Job drawing, mm, ordinate dimensions from the low corner. One solid piece. A direction names the side the tool comes from. Round coordinates to 2 decimals unless told otherwise and drop trailing zeros. Loops run counter-clockwise (first coordinate to the right, second up) from the corner with the lowest first, then second, coordinate; pieces in that order, holes last. Notation, with made-up numbers: M 34.5,62.5 L 39.5,62.5 A36 ccw 39.5,99.5 Z; hole C 13,17.5 d11. An arc over 180 degrees is marked long. Use a Markdown table: item, result. Add a question column.
(1) Flat gauge pins, fed straight in: P1, Ø4, axis at x = 19.5, z = 8, coming from the +Y side; P2, Ø2, axis at y = 6, z = 11.5, coming from the +X side; P3, Ø3, axis at x = 25, z = 10.5, coming from the +Y side; P4, Ø1.5, axis at x = 30, z = 9.5, coming from the -Y side. Where does each tip first touch, or does it go through?
(2) Which spindle directions (+Z, -Z, +X, -X, +Y, -Y) get a long thin tool onto all of the face, cutting with end or side? Do the marked faces 1, 2, 3 and 4. Say none if no direction does.
(3) Band-saw the part on A-A, the plane z = 3.75. Write the cut outline in (x, y).
(4) Band-saw the part on B-B, the plane y = 19.75. Write the cut outline in (x, z).
(5) Wall check: L1, parallel to Y at x = 12, z = 10.25; L2, parallel to X at y = 4.5, z = 1.75; L3, parallel to Y at x = 30, z = 2.75. Give the ranges that are in metal, low to high.
(6) Band-saw the part on D-D, the plane z = 6.5. Write the cut outline in (x, y).
(7) Band-saw the part on C-C, the plane x = 30. Write the cut outline in (y, z), and give its area (3 significant figures).
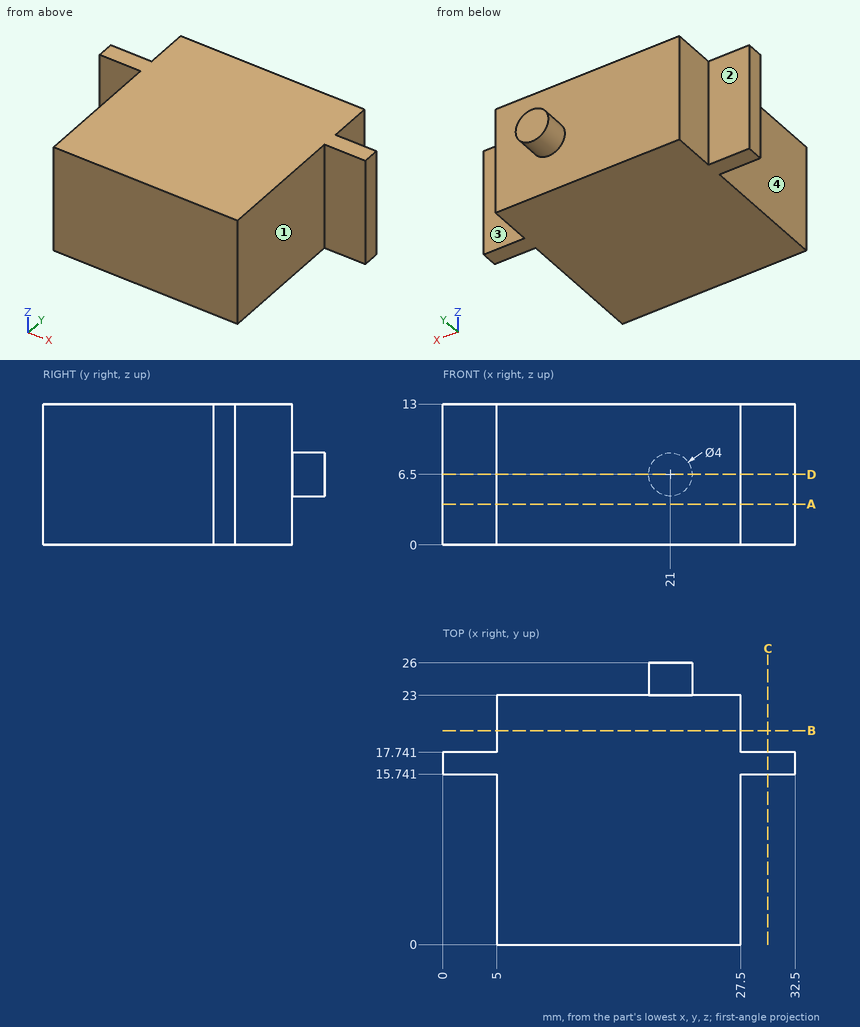
Return value:
| question | item | result |
|---|---|---|
| 1 | P1 | y = 26 |
| 1 | P2 | x = 27.5 |
| 1 | P3 | y = 23 |
| 1 | P4 | y = 15.74 |
| 2 | face 1 | +Z, -Z, +X, -Y |
| 2 | face 2 | +Z, -Z, -X, +Y |
| 2 | face 3 | +Z, -Z, +X, +Y |
| 2 | face 4 | +Z, -Z, -X, -Y |
| 3 | outline | M 0,15.74 L 5,15.74 L 5,0 L 27.5,0 L 27.5,15.74 L 32.5,15.74 L 32.5,17.74 L 27.5,17.74 L 27.5,23 L 5,23 L 5,17.74 L 0,17.74 Z |
| 4 | outline | M 5,0 L 27.5,0 L 27.5,13 L 5,13 Z |
| 5 | L1 | 0 to 23 |
| 5 | L2 | 5 to 27.5 |
| 5 | L3 | 15.74 to 17.74 |
| 6 | outline | M 0,15.74 L 5,15.74 L 5,0 L 27.5,0 L 27.5,15.74 L 32.5,15.74 L 32.5,17.74 L 27.5,17.74 L 27.5,23 L 23,23 L 23,26 L 19,26 L 19,23 L 5,23 L 5,17.74 L 0,17.74 Z |
| 7 | outline | M 15.74,0 L 17.74,0 L 17.74,13 L 15.74,13 Z |
| 7 | area | 26.0 mm^2 |
